Could you check a few things on this model? Use its own coordinates, in mm. Face numbers are marked on the shaded views. Give positions to 0.01 mm unless a question says otherwise; leave off trailing zeros. Loops run counter-clockwise (first coordinate to the right, second up) from the corner with the lowest first, then second, coordinate; pieces in that order, holes last. Notation, with made-up numbers: (56.5, 8.5) - (91.5, 8.5) arc R12 ccw to (91.5, 19.5) - close; hole circle Ø4 at (68.5, 88). An arc over 180 degrees is marked (long way). One line per item, written item: value. Start each with the question number.
Q1. I want a section at D-D (z = 105). Please give me the cut outline in (x, y), then the cut area to 3 significant figures.
Q2. I'm going to push flat-ended pins straight in: P1, Ø10, axis at x = 26, y = 3, coming from the +Z side; P2, Ø6.5, axis at x = 50, y = -50, coming from the -Z side; P3, Ø10, axis at x = -35, y = 36.5, coming from the -Z side. Where does each tip first touch, or does it pass through?
Q3. I want a section at B-B (x = -4). Please give me the cut outline in (y, z).
Q4. If I drill on line 1 (X direction, y = -50, z = 121.5); line 2 (X direction, y = 51, z = 114); line 3 (Y direction, x = 0, z = 106.75), over which ranges is the centre line in solid material (lowest first)? Write a range as from..to.
Q5. If we mould it in two halves opening along Y, with no side actions, what happens to the marked faces 1, 2, 3 and 4? For each: released by +Y, released by -Y, zero draft, split by the parting line, or undercut.
Q6. I want a section at A-A (z = 117.5). Please give me the cut outline in (x, y), then the cut area to 3 significant figures.
Q7. I want a section at C-C (y = -21). Please give me the cut outline in (x, z), then the cut area to 3 significant figures.
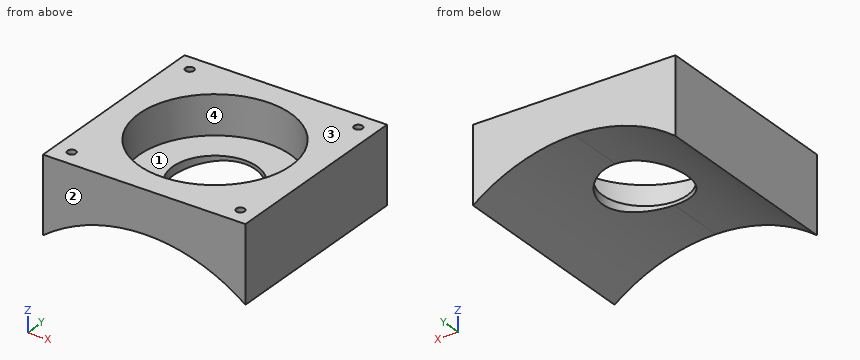
```python
from build123d import *

# Parameters (mm, degrees)
F1_DEPTH = 60
F2_R     = 25
F3_DEPTH = 50
F4_R     = 45
F5_DEPTH = 23
F7_D     = 5
F7_DEPTH = 15
F7_TIP   = 1.5021515476


with BuildPart() as f1:
    # F0 (on Front) → F1 (new body, symmetric)
    with BuildSketch(Plane.XZ):
        with BuildLine():
            ThreePointArc((0, 100), (31.6227766017, 94.8683298051), (60, 80))
            Line((60, 80), (60, 125))
            Line((60, 125), (-60, 125))
            Line((-60, 125), (-60, 80))
            ThreePointArc((-60, 80), (-31.6227766017, 94.8683298051), (0, 100))
        make_face()
    extrude(amount=F1_DEPTH, both=True)

    # F2 (on face) → F3 (cut)
    with BuildSketch(Plane.XY.offset(125)):
        Circle(F2_R)
    extrude(amount=-F3_DEPTH, mode=Mode.SUBTRACT)

    # F4 (on face) → F5 (cut)
    with BuildSketch(Plane.XY.offset(125)):
        Circle(F4_R)
    extrude(amount=-F5_DEPTH, mode=Mode.SUBTRACT)

    # F7
    with Locations(Plane.XY.offset(125)):
        with Locations((-50, 50), (50, 50), (50, -50), (-50, -50)):
            Hole(F7_D / 2, depth=F7_DEPTH)
            with Locations((0, 0, -(F7_DEPTH + F7_TIP / 2))):  # 118° drill point
                Cone(0, F7_D / 2, F7_TIP, mode=Mode.SUBTRACT)


solid = f1.part
```
Worked answers:
1. outline: (-60, -60) - (60, -60) - (60, 60) - (-60, 60) - close; hole circle Ø90 at (0, 0)
1. area: 8,040 mm²
2. P1: stops at z = 102
2. P2: stops at z = 84.64
2. P3: stops at z = 91.65
3. outline: (-60, 99.92) - (-24.68, 99.92) - (-24.68, 102) - (-44.82, 102) - (-44.82, 125) - (-60, 125) - close; (24.68, 99.92) - (60, 99.92) - (60, 125) - (44.82, 125) - (44.82, 102) - (24.68, 102) - close
4. line 1: x = -60..-52.5, -47.5..47.5, 52.5..60
4. line 2: x = -60..-52.29, -47.71..47.71, 52.29..60
4. line 3: y = -60..-45, 45..60
5. face 1: undercut
5. face 2: released by -Y
5. face 3: zero draft
5. face 4: undercut
6. outline: (-60, -60) - (60, -60) - (60, 60) - (-60, 60) - close; hole circle Ø5 at (-50, -50); hole circle Ø5 at (-50, 50); hole circle Ø90 at (0, 0); hole circle Ø5 at (50, -50); hole circle Ø5 at (50, 50)
6. area: 7,960 mm²
7. outline: (-60, 80) arc R100 cw to (-13.56, 99.08) - (-13.56, 102) - (-39.8, 102) - (-39.8, 125) - (-60, 125) - close; (13.56, 99.08) arc R100 cw to (60, 80) - (60, 125) - (39.8, 125) - (39.8, 102) - (13.56, 102) - close
7. area: 1,870 mm²
